from build123d import *

# Parameters (mm, degrees)
SKETCH1_W           = 7.2
SKETCH1_H           = 12
BOSS_EXTRUDE1_DEPTH = 2
SKETCH2_W           = 10
SKETCH2_H           = 24
BOSS_EXTRUDE2_DEPTH = 6
CUT_EXTRUDE1_DEPTH  = 24


with BuildPart() as part:
    # Sketch1 → Boss-Extrude1 (new body)
    with BuildSketch(Plane.XY):
        Rectangle(SKETCH1_W, SKETCH1_H)
    extrude(amount=BOSS_EXTRUDE1_DEPTH)

    # Sketch2 → Boss-Extrude2 (add)
    with BuildSketch(Plane.XY.offset(2)):
        with Locations((0, 6)):
            Rectangle(SKETCH2_W, SKETCH2_H)
    extrude(amount=BOSS_EXTRUDE2_DEPTH)

    # Sketch5 → Cut-Extrude1 (cut)
    with BuildSketch(Plane(origin=(0, 18, 0), x_dir=(1, 0, 0), z_dir=(0, 1, 0))):
        with BuildLine():
            Line((-4, -8), (4, -8))
            ThreePointArc((4, -8), (0, -4), (-4, -8))
        make_face()
    extrude(amount=-CUT_EXTRUDE1_DEPTH, mode=Mode.SUBTRACT)


solid = part.part
Design review of the part built by this model. Coordinates are the model's own, in mm. A direction names the side the tool comes from. Give positions to 0.01 mm unless a question says otherwise; leave off trailing zeros. Loops run counter-clockwise (first coordinate to the right, second up) from the corner with the lowest first, then second, coordinate; pieces in that order, holes last. Notation, with made-up numbers: (55, 13) -> (105, 13) arc R15 cw to (105, 19) -> close; hole circle Ø10 at (53.5, -3). An arc over 180 degrees is marked (long way). One line per question, with ' | ' between items. Start each with the question number.
(1) We need section B-B (y = -1.75). State the section outline as (x, z) points, and give its area (3 significant figures).
(2) We need section D-D (z = 5.5). State the section outline as (x, y) points.
(3) For line 1 (X direction, y = 2.75, z = 7.5); line 2 (X direction, y = 5.75, z = 5.75); line 3 (Y direction, x = 2, z = 1.25), list the stretches that pass through material, from the lowest coordinate up.
(4) Draft analysis for pull direction Y (two halves, no side actions). For faces 1 (the face through (0, -6, 3)), 2 (the face through (0, 6, 1)), 3 (the face through (-5, 6, 5)), state which applies: +Y half, -Y half, draft (parallel to the pull), parting line (faces both ways), or undercut.
(5) We need section C-C (x = 4.75). State the section outline as (y, z) points.
(6) Insertion check: P1, Ø2, axis at x = -0.5, z = 1.5, coming from the +Y side; P2, Ø5, axis at x = -2.5, y = 9.5, coming from the -Z side; P3, Ø1.6, axis at x = 0.5, z = 1, coming from the +Y side; P4, Ø1.6, axis at y = 2.5, z = 0.5, coming from the -X side. Each pin has a flat end and moves straight along its axis. Give the tip position at first contact, or say it passes through.
(7) We need section A-A (z = 7.5). State the section outline as (x, y) points.
(8) For faces 4 (the face through (-3.6, 0, 1)), 5 (the face through (3.6, 0, 1)), 6 (the face through (-0.1, 18, 3.6)), list the 3-axis set-ups (+Z, -Z, +X, -X, +Y, -Y) from which the entire face can be reached by the end or side of a thin tool; tool diameter is ignored.
The answers:
1) outline: (-5, 2) -> (-3.6, 2) -> (-3.6, 0) -> (3.6, 0) -> (3.6, 2) -> (5, 2) -> (5, 8) -> (4, 8) arc R4 cw to (-4, 8) -> (-5, 8) -> close | area: 49.3 mm^2
2) outline: (-5, -6) -> (-3.12, -6) -> (-3.12, 18) -> (-5, 18) -> close; (3.12, -6) -> (5, -6) -> (5, 18) -> (3.12, 18) -> close
3) line 1: x = -5 to -3.97, 3.97 to 5 | line 2: x = -5 to -3.31, 3.31 to 5 | line 3: y = -6 to 6
4) face 1: -Y half | face 2: +Y half | face 3: draft
5) outline: (-6, 2) -> (18, 2) -> (18, 8) -> (-6, 8) -> close
6) P1: stops at y = 18 | P2: stops at z = 2 | P3: stops at y = 6 | P4: stops at x = -3.6
7) outline: (-5, -6) -> (-3.97, -6) -> (-3.97, 18) -> (-5, 18) -> close; (3.97, -6) -> (5, -6) -> (5, 18) -> (3.97, 18) -> close
8) face 4: -Z, -X, +Y, -Y | face 5: -Z, +X, +Y, -Y | face 6: +Z, -Z, +X, -X, +Y
